Input: dimensioned drawing with shaded views. Units: mm. Origin: part minimum x, y, z. A direction names the side the tool comes from. Round coordinates to 2 decimals unless told otherwise and drop trailing zeros. Order: outer loops, then holes, each group sorted by start corner. A loop starts at its lowest first (then second) coordinate and runs counter-clockwise, first axis right, second up. Notation, with made-up numbers: (38.25, 44.25) - (81.25, 44.25) arc R18 ccw to (81.25, 51.25) - close; hole circle Ø9 at (-6, 6). An arc over 180 degrees is marked (long way). One line per item, written item: value. Start each with the question number.
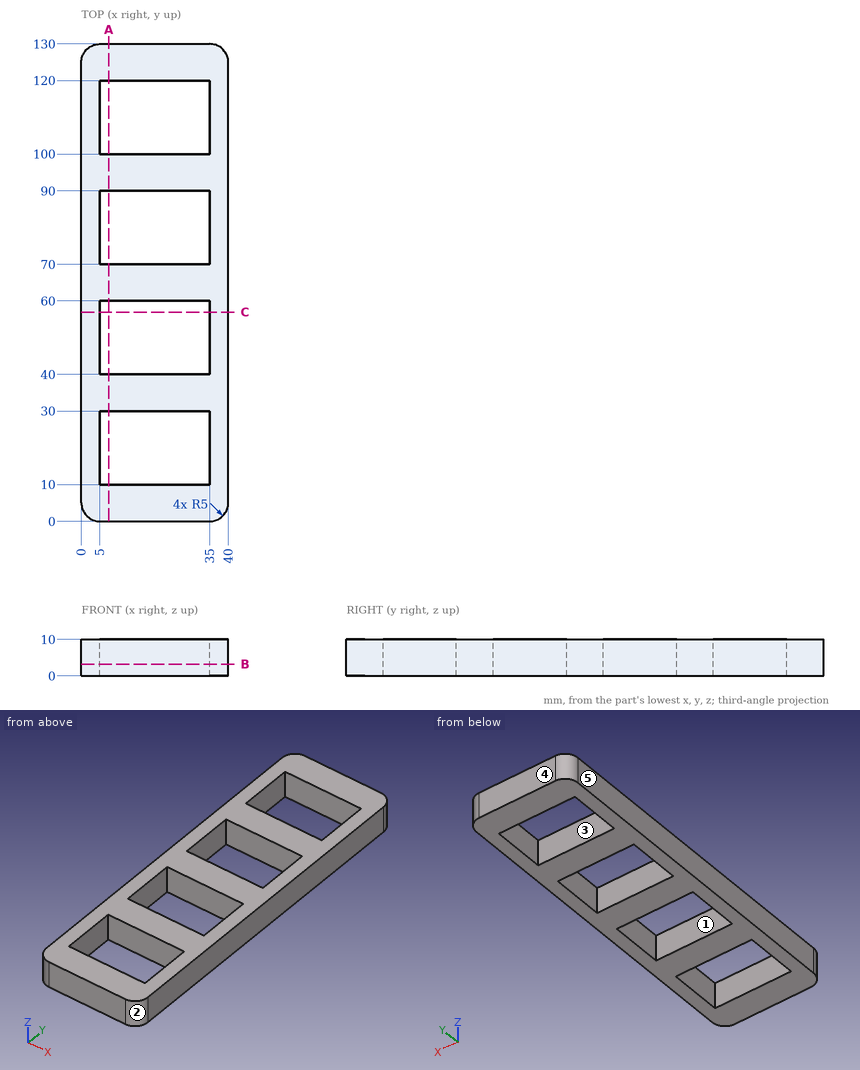
1. Line query: line 1 (Y direction, x = 14.5, z = 6.5); line 2 (X direction, y = 21, z = 4.75); line 3 (Y direction, x = 35.5, z = 9.5). Output: solid intervals per line, ascending. Write a range as from..to.
2. Section A-A (x = 7.5). Return the cut outline in (y, z), then the cut area to 3 significant figures.
3. Pin query (flat end, axial travel): pin 1 (2 mm diameter, centred on y = 70, z = 5.5, fed in from -X). Return the tip coordinate at first contact, or that it passes through.
4. Pull-direction query (Y, two-part tool) for the marked faces 3, 4 and 5; classes: released by +Y, released by -Y, zero draft, split by the parting line, or undercut.
5. Section B-B (z = 3.25). Return the cut outline in (x, y), then the cut area to 3 significant figures.
6. Section C-C (y = 57). Return the cut outline in (x, z), then the cut area to 3 significant figures.
7. Set-up query: the marked faces 1 and 2. Return all of +Z, -Z, +X, -X, +Y, -Y with unobstructed straight access to the full face (end or side cutting, diameter ignored); none if empty.
Solved:
1. line 1: y = 0..10, 30..40, 60..70, 90..100, 120..130
1. line 2: x = 0..5, 35..40
1. line 3: y = 0.03..129.97
2. outline: (0, 0) - (10, 0) - (10, 10) - (0, 10) - close; (30, 0) - (40, 0) - (40, 10) - (30, 10) - close; (60, 0) - (70, 0) - (70, 10) - (60, 10) - close; (90, 0) - (100, 0) - (100, 10) - (90, 10) - close; (120, 0) - (130, 0) - (130, 10) - (120, 10) - close
2. area: 500 mm²
3. pin 1: stops at x = 0
4. face 3: undercut
4. face 4: released by +Y
4. face 5: zero draft
5. outline: (0, 5) arc R5 ccw to (5, 0) - (35, 0) arc R5 ccw to (40, 5) - (40, 125) arc R5 ccw to (35, 130) - (5, 130) arc R5 ccw to (0, 125) - close; hole (5, 10) - (35, 10) - (35, 30) - (5, 30) - close; hole (5, 40) - (35, 40) - (35, 60) - (5, 60) - close; hole (5, 70) - (35, 70) - (35, 90) - (5, 90) - close; hole (5, 100) - (35, 100) - (35, 120) - (5, 120) - close
5. area: 2,780 mm²
6. outline: (0, 0) - (5, 0) - (5, 10) - (0, 10) - close; (35, 0) - (40, 0) - (40, 10) - (35, 10) - close
6. area: 100 mm²
7. face 1: +Z, -Z
7. face 2: +Z, -Z, +X, -Y
